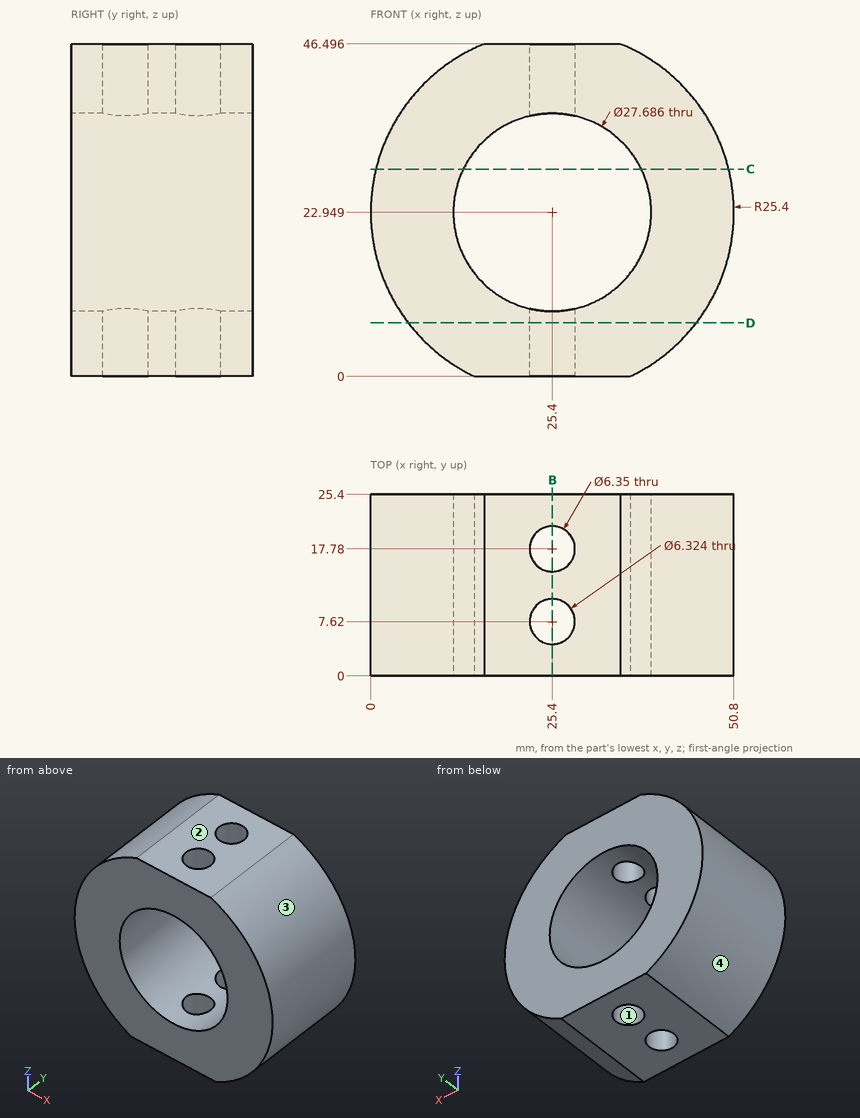
Source: three-view drawing plus pictorial views. Frame: mm from the lowest corner of the part. Coordinates: 2 decimals unless noted, no trailing zeros. Loops run counter-clockwise (first coordinate to the right, second up) from the corner with the lowest first, then second, coordinate; pieces in that order, holes last. Notation, with made-up numbers: (82.5, -16.5) -> (102.5, -16.5) arc R19 cw to (102.5, 20.5) -> close; hole circle Ø10 at (71.5, -26). An arc over 180 degrees is marked (long way). Write each question's results on one line, items separated by ' | '. Start each with the question number.
Q1. Ray query, line 1 (Y direction, x = 25.4, z = 5) (1 decimal); line 2 (Z direction, x = 25, y = 11.5) (1 decimal); line 3 (X direction, y = 3.75, z = 22). Return the intervals inside material, ascending. Write a range as from..to.
Q2. Pull-direction query (X, two-part tool) for the marked faces 1, 2, 3 and 4; classes: released by +X, released by -X, zero draft, split by the parting line, or undercut.
Q3. Section C-C, the plane z = 29. Return the cut outline in (x, y).
Q4. Pin query (flat end, axial travel): pin 1 (5.5 mm diameter, centred on x = 25.4, y = 17.78, fed in from +Z); pin 2 (2 mm diameter, centred on y = 17, z = 21.5, fed in from +X); pin 3 (4 mm diameter, centred on x = 8.5, y = 21.5, fed in from +Z); pin 4 (10 mm diameter, centred on y = 20.5, z = 9.5, fed in from +X). Return the tip coordinate at first contact, or that it passes through.
Q5. Section B-B, the plane x = 25.4. Return the cut outline in (y, z) (1 decimal).
Q6. Section D-D, the plane z = 7.5. State how many separate pieces and enclosed holes the cut face has, plus the area to 3 significant figures.
Found:
1) line 1: 0..4.5, 10.8..14.6, 21..25.4 | line 2: 0..9.1, 36.8..46.5 | line 3: 0.02..11.59, 39.21..50.78
2) face 1: undercut | face 2: zero draft | face 3: released by +X | face 4: released by -X
3) outline: (0.73, 0) -> (12.95, 0) -> (12.95, 25.4) -> (0.73, 25.4) -> close; (37.85, 0) -> (50.07, 0) -> (50.07, 25.4) -> (37.85, 25.4) -> close
4) pin 1: through | pin 2: x = 50.8 | pin 3: z = 43.52 | pin 4: x = 49.35
5) outline: (0, 0) -> (4.5, 0) -> (4.5, 9.1) -> (0, 9.1) -> close; (0, 36.8) -> (4.5, 36.8) -> (4.5, 46.5) -> (0, 46.5) -> close; (10.8, 0) -> (14.6, 0) -> (14.6, 9.1) -> (10.8, 9.1) -> close; (10.8, 36.8) -> (14.6, 36.8) -> (14.6, 46.5) -> (10.8, 46.5) -> close; (21, 0) -> (25.4, 0) -> (25.4, 9.1) -> (21, 9.1) -> close; (21, 36.8) -> (25.4, 36.8) -> (25.4, 46.5) -> (21, 46.5) -> close
6) separate pieces: 1 | enclosed holes: 2 | area: 961 mm2
